Here's the drawing with two shaded views (mm, measured from the low corner). I have some questions. Coordinates: 2 decimals unless noted, no trailing zeros. Order: outer loops, then holes, each group sorted by start corner. A loop starts at its lowest first (then second) coordinate and runs counter-clockwise, first axis right, second up. Notation, with made-up numbers: (-10.5, -36) -> (19.5, -36) arc R9 ccw to (19.5, -19) -> close; hole circle Ø6 at (81.5, 7). An arc over 180 degrees is marked (long way). Answer as a JSON object with one key per item and string values. Group by question number.
(1) I want a section at A-A, the plane x = 52.5. List the corners of the cut face in (y, z) for me, plus the area to 3 significant figures.
(2) If we mould it in two halves opening along X, with no side actions, what happens to the marked faces 1, 2 and 3? For each: pulls with the +X half, pulls with the -X half, needs draft (parallel to the pull), parting line crosses it, or undercut.
(3) I need wall thicknesses on line 1 (Y direction, x = 17.5, z = 2.5); line 2 (X direction, y = 8.5, z = 6.5); line 3 (X direction, y = 7, z = 6.5). Which ranges of each line are inside material? Lowest first, please.
(4) I want a section at C-C, the plane y = 10. List the corners of the cut face in (x, z) for me.
(5) For pin 1 (4 mm diameter, centred on x = 33.5, z = 4.5, fed in from -Y), with a flat end and sliding along its axis, tell me the tip position at first contact or that it passes through.
(6) I want a section at B-B, the plane z = 8.25. List the corners of the cut face in (x, y) for me.
(7) I want a section at D-D, the plane x = 19.5. List the corners of the cut face in (y, z) for me.
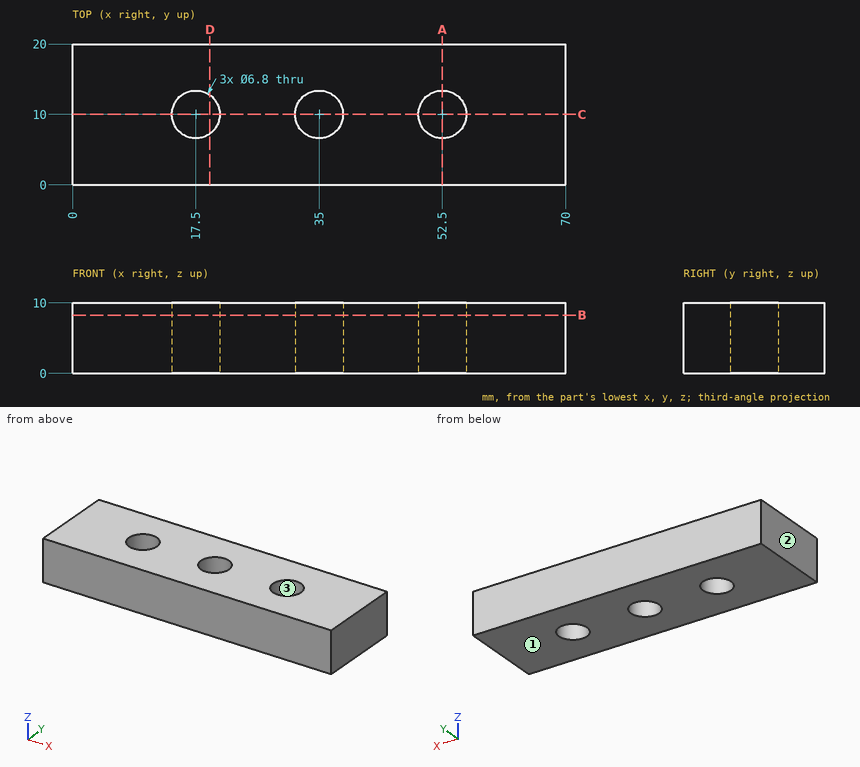
Computed values:
{
 "1": {"outline": "(0, 0) -> (6.6, 0) -> (6.6, 10) -> (0, 10) -> close; (13.4, 0) -> (20, 0) -> (20, 10) -> (13.4, 10) -> close", "area": "132 mm2"},
 "2": {"face 1": "needs draft", "face 2": "pulls with the -X half", "face 3": "undercut"},
 "3": {"line 1": "y = 0 to 6.6, 13.4 to 20", "line 2": "x = 0 to 14.45, 20.55 to 31.95, 38.05 to 49.45, 55.55 to 70", "line 3": "x = 0 to 15.9, 19.1 to 33.4, 36.6 to 50.9, 54.1 to 70"},
 "4": {"outline": "(0, 0) -> (14.1, 0) -> (14.1, 10) -> (0, 10) -> close; (20.9, 0) -> (31.6, 0) -> (31.6, 10) -> (20.9, 10) -> close; (38.4, 0) -> (49.1, 0) -> (49.1, 10) -> (38.4, 10) -> close; (55.9, 0) -> (70, 0) -> (70, 10) -> (55.9, 10) -> close"},
 "5": {"pin 1": "stops at y = 0"},
 "6": {"outline": "(0, 0) -> (70, 0) -> (70, 20) -> (0, 20) -> close; hole circle Ø6.8 at (17.5, 10); hole circle Ø6.8 at (35, 10); hole circle Ø6.8 at (52.5, 10)"},
 "7": {"outline": "(0, 0) -> (7.25, 0) -> (7.25, 10) -> (0, 10) -> close; (12.75, 0) -> (20, 0) -> (20, 10) -> (12.75, 10) -> close"}
}
